from build123d import *

# Parameters (mm, degrees)
BOSS_EXTRUDE1_DEPTH = 5.715
BOSS_EXTRUDE2_DEPTH = 6.6675
BOSS_EXTRUDE3_START = 6.6675
BOSS_EXTRUDE3_DEPTH = 6.6675
FILLET1_R           = 2.54
SKETCH5_R           = 1.524
CUT_EXTRUDE1_DEPTH  = 6.35
SKETCH6_W           = 6.0325
SKETCH6_H           = 6.096
CUT_EXTRUDE2_DEPTH  = 110.257060148
SKETCH7_W           = 13.176307298
SKETCH7_H           = 9.310122243
CUT_EXTRUDE3_DEPTH  = 110.257060009


with BuildPart() as part:
    # Sketch1 → Boss-Extrude1 (new body)
    with BuildSketch(Plane.XY):
        with BuildLine():
            ThreePointArc((69.342, 76.073), (0, 6.731), (-69.342, 76.073))
            Line((-69.342, 76.073), (-76.073, 76.073))
            ThreePointArc((-76.073, 76.073), (0, 0), (76.073, 76.073))
            Line((76.073, 76.073), (69.342, 76.073))
        make_face()
    extrude(amount=BOSS_EXTRUDE1_DEPTH)

    # Sketch3 → Boss-Extrude2 (add)
    with BuildSketch(Plane.XY.offset(5.715)):
        with BuildLine():
            ThreePointArc((65.5955, 76.073), (0, 10.4775), (-65.5955, 76.073))
            Line((-65.5955, 76.073), (-69.342, 76.073))
            ThreePointArc((-69.342, 76.073), (0, 6.731), (69.342, 76.073))
            Line((69.342, 76.073), (65.5955, 76.073))
        make_face()
        with BuildLine():
            Line((76.073, 76.073), (69.342, 76.073))
            ThreePointArc((69.342, 76.073), (0, 6.731), (-69.342, 76.073))
            Line((-69.342, 76.073), (-76.073, 76.073))
            ThreePointArc((-76.073, 76.073), (0, 0), (76.073, 76.073))
        make_face()
    extrude(amount=BOSS_EXTRUDE2_DEPTH)

    # Sketch4 → Boss-Extrude3 (add)
    with BuildSketch(Plane(origin=(0, 0, 0), x_dir=(-1, 0, 0), z_dir=(0, 0, -1)).offset(BOSS_EXTRUDE3_START)):
        with BuildLine():
            ThreePointArc((65.5955, 76.073), (0, 10.4775), (-65.5955, 76.073))
            Line((-65.5955, 76.073), (-69.342, 76.073))
            ThreePointArc((-69.342, 76.073), (0, 6.731), (69.342, 76.073))
            Line((69.342, 76.073), (65.5955, 76.073))
        make_face()
        with BuildLine():
            Line((76.073, 76.073), (69.342, 76.073))
            ThreePointArc((69.342, 76.073), (0, 6.731), (-69.342, 76.073))
            Line((-69.342, 76.073), (-76.073, 76.073))
            ThreePointArc((-76.073, 76.073), (0, 0), (76.073, 76.073))
        make_face()
    extrude(amount=-BOSS_EXTRUDE3_DEPTH)

    # Fillet1
    fillet1_edges = [part.edges().sort_by_distance(p)[0] for p in [
        (0, 6.731, 5.715),
        (0, 6.731, 0),
    ]]
    fillet(fillet1_edges, radius=FILLET1_R)

    # Sketch5 → Cut-Extrude1 (cut)
    with BuildSketch(Plane(origin=(0, 0, 0), x_dir=(1, 0, 0), z_dir=(0, 1, 0))):
        with Locations(Location((0, -2.8575, 0), (0, 0, 90))):
            Circle(SKETCH5_R)
    extrude(amount=CUT_EXTRUDE1_DEPTH, mode=Mode.SUBTRACT)

    # Sketch6 → Cut-Extrude2 (cut, through all)
    with BuildSketch(Plane.XY.offset(12.3825)):
        with BuildLine():
            Line((-82.07762594, 69.977), (-75.828359556, 69.977))
            ThreePointArc((-75.828359556, 69.977), (-76.011815284, 73.022546552), (-76.073, 76.073))
            Line((-76.073, 76.073), (-82.07762594, 76.073))
            Line((-82.07762594, 76.073), (-82.07762594, 69.977))
        make_face()
        with Locations((-72.812109556, 73.025)):
            Rectangle(SKETCH6_W, SKETCH6_H)
        with BuildLine():
            ThreePointArc((76.073, 76.073), (76.011815284, 73.022546552), (75.828359556, 69.977))
            Line((75.828359556, 69.977), (82.07762594, 69.977))
            Line((82.07762594, 69.977), (82.07762594, 76.073))
            Line((82.07762594, 76.073), (76.073, 76.073))
        make_face()
        with Locations((72.812109556, 73.025)):
            Rectangle(SKETCH6_W, SKETCH6_H)
    extrude(amount=-CUT_EXTRUDE2_DEPTH, mode=Mode.SUBTRACT)


with BuildPart() as cut_extrude2_piece_1:
    # of the separate pieces the step leaves, piece 1, a body of its own (cut_extrude2_pieces)
    add(part.part.solids().sort_by_distance((66.802, 76.073, 5.715))[0])


with BuildPart() as cut_extrude2_piece_2:
    # of the separate pieces the step leaves, piece 2, a body of its own (cut_extrude2_pieces)
    add(part.part.solids().sort_by_distance((75.828359556, 76.073, 12.3825))[0])


with BuildPart() as cut_extrude2_piece_3:
    # of the separate pieces the step leaves, piece 3, a body of its own (cut_extrude2_pieces)
    add(part.part.solids().sort_by_distance((-76.073, 76.073, 12.3825))[0])


with BuildPart() as cut_extrude3_tool:
    # Sketch7 → Cut-Extrude3 (new, through all)
    with BuildSketch(Plane.XY.offset(12.3825)):
        with Locations((-79.400263205, 74.632061122)):
            Rectangle(SKETCH7_W, SKETCH7_H)
        with Locations((79.400263205, 74.632061122)):
            Rectangle(SKETCH7_W, SKETCH7_H)
    extrude(amount=-CUT_EXTRUDE3_DEPTH)


with BuildPart() as cut_extrude2_piece_2_1:
    add(cut_extrude2_piece_2.part)

    # Cut-Extrude3: cut by cut_extrude3_tool
    add(cut_extrude3_tool.part, mode=Mode.SUBTRACT)


with BuildPart() as cut_extrude2_piece_3_1:
    add(cut_extrude2_piece_3.part)

    # Cut-Extrude3: cut by cut_extrude3_tool
    add(cut_extrude3_tool.part, mode=Mode.SUBTRACT)


solid = cut_extrude2_piece_1.part
Can you work these out from the model? Positions are in its coordinate system, mm. A direction names the side the tool comes from. Give positions to 0.01 mm unless a question says otherwise; leave off trailing zeros. Loops run counter-clockwise (first coordinate to the right, second up) from the corner with the lowest first, then second, coordinate; pieces in that order, holes last. Notation, with made-up numbers: (37.5, -0.75) - (69.5, -0.75) arc R25 ccw to (69.5, 29.25) - close; hole circle Ø4 at (47.25, -21.75). An arc over 180 degrees is marked (long way). Return JSON: item names as keys, results as strings.
1. If I drill on line 1 (X direction, y = 65, z = -3); line 2 (X direction, y = 47, z = 10.75); line 3 (Z direction, x = -44, y = 24), over which ranges is the centre line in solid material (lowest first)?
Output values:
{"line 1": "x = -75.26 to -64.65, 64.65 to 75.26", "line 2": "x = -70.3 to -58.8, 58.8 to 70.3", "line 3": "z = -6.67 to 0.4, 5.31 to 12.38"}
2. For faces 5 (the face through (0.58, 3.13, 1.45)), 6 (the face through (-10, 11, 5.715)), 7 (the face through (-69.796, 73, 3)), 8 (the face through (69.796, 73, 3)), which set-ups out of +Z, -Z, +X, -X, +Y, -Y let a thin tool reach every point of the face, with its end or its side?
Output values:
{"face 5": "-Y", "face 6": "+Y", "face 7": "+Z, -Z, -X, +Y", "face 8": "+Z, -Z, +X, +Y"}
3. I want a section at B-B on z = 8. Please give me the cut outline in (x, y).
Output values:
{"outline": "(-75.83, 69.98) arc R76.07 ccw to (75.83, 69.98) - (69.8, 69.98) - (69.8, 76.07) - (65.6, 76.07) arc R65.6 cw to (-65.6, 76.07) - (-69.8, 76.07) - (-69.8, 69.98) - close"}
4. I'm going to push flat-ended pins straight in: pin 1 Ø1 at (x, z) = (-27.5, -1) entering from +Y; pin 2 Ø6 at (y, z) = (32, 10.5) entering from +X; pin 3 Ø3 at (x, z) = (53.5, 6) entering from -Y; pin 4 Ø5 at (y, z) = (72, 5.5) entering from +X. Where does each tip first touch, or does it pass through?
Output values:
{"pin 1": "stops at y = 16.75", "pin 2": "stops at x = 64.03", "pin 3": "stops at y = 20.55", "pin 4": "stops at x = 75.83"}
5. We'd pull the mould along Z, two halves only. Please class faces 1 (the face through (0, 10, -6.668)), 2 (the face through (73, 69.977, 3)), 3 (the face through (0, 6.35, 3)), 4 (the face through (0, 10, 12.382)): +Z half, -Z half, draft (parallel to the pull), parting line (faces both ways), or undercut.
Output values:
{"face 1": "-Z half", "face 2": "draft", "face 3": "undercut", "face 4": "+Z half"}
